Input: part model. Units: mm. Frame: model coordinates. A direction names the side the tool comes from. Give positions to 0.01 mm unless a question says otherwise; leave off trailing zeros. Order: outer loops, then holes, each group sorted by start corner. A loop starts at its lowest first (then second) coordinate and runs counter-clockwise, first axis right, second up. Notation, with made-up numbers: (89, 69) - (142, 69) arc R15 cw to (142, 91) - close; hole circle Ø8 at (57.25, -38). An arc over 180 degrees is marked (long way). Answer in a Markdown table with one row per item. Add a question column.
1. Section query B-B on y = -74. Return loops of the section in (x, z).
2. Contact query for flat-ended pins moving along their axis: pin 1 (1.5 mm diameter, centred on y = -72, z = 32.5, fed in from +X); pin 2 (4 mm diameter, centred on x = 160, z = 63.5, fed in from +Y); pin 3 (2 mm diameter, centred on x = 156, z = 37, fed in from +Y). Output: stop coordinate, or through.
3. Ray query, line 1 (X direction, y = -99.5, z = 61); line 2 (Y direction, x = -151.5, z = 40); line 3 (Y direction, x = 164, z = 22.5). Return the intervals inside material, ascending. Write a range as [from, to].
4. Section query C-C on y = 5.5. Return loops of the section in (x, z), and give its area (3 significant figures).
5. Section query A-A on z = 52.5. Return loops of the section in (x, y).
6. Access query for faces 1 (the face through (149.627, -57, 42)), 2 (the face through (-149.627, -49, 42)), 3 (the face through (-199.22, 64.44, 42.4)). Directions: +Z, -Z, +X, -X, +Y, -Y. A direction counts if a zero-diameter tool reaches every point of the face in a straight line with its end or side. Return the directions, or none.
```python
from build123d import *

# Parameters (mm, degrees)
F1_DEPTH = 86.007776


with BuildPart() as f1:
    # F0 (on Top) → F1 (new body)
    with BuildSketch(Plane.XY):
        Polygon((149.626926, 0), (149.626926, 112.95262), (-149.626926, 112.95262), (-149.626926, 13.745412), (-149.626926, -112.95262), (149.626926, -112.95262), align=None)
        with BuildLine():
            Line((-149.626926, 13.745412), (-149.626926, 112.95262))
            ThreePointArc((-149.626926, 112.95262), (-199.230529, 63.349016), (-149.626926, 13.745412))
        make_face()
        with BuildLine():
            ThreePointArc((149.626926, 0), (206.103235, 56.47631), (149.626926, 112.95262))
            Line((149.626926, 112.95262), (149.626926, 0))
        make_face()
    extrude(amount=F1_DEPTH)


solid = f1.part
```
Answer:
| question | item | result |
|---|---|---|
| 1 | outline | (-149.63, 0) - (149.63, 0) - (149.63, 86.01) - (-149.63, 86.01) - close |
| 2 | pin 1 | stops at x = 149.63 |
| 2 | pin 2 | stops at y = 112.33 |
| 2 | pin 3 | stops at y = 112.7 |
| 3 | line 1 | x = [-149.63, 149.63] |
| 3 | line 2 | y = [13.78, 112.92] |
| 3 | line 3 | y = [1.86, 111.09] |
| 4 | outline | (-149.63, 0) - (173.94, 0) - (173.94, 86.01) - (-149.63, 86.01) - close |
| 4 | area | 27,800 mm² |
| 5 | outline | (-149.63, -112.95) - (149.63, -112.95) - (149.63, 0) arc R56.48 ccw to (149.63, 112.95) - (-149.63, 112.95) arc R49.6 ccw to (-149.63, 13.75) - close |
| 6 | face 1 | +Z, -Z, +X, -Y |
| 6 | face 2 | +Z, -Z, -X, -Y |
| 6 | face 3 | +Z, -Z, -X |
